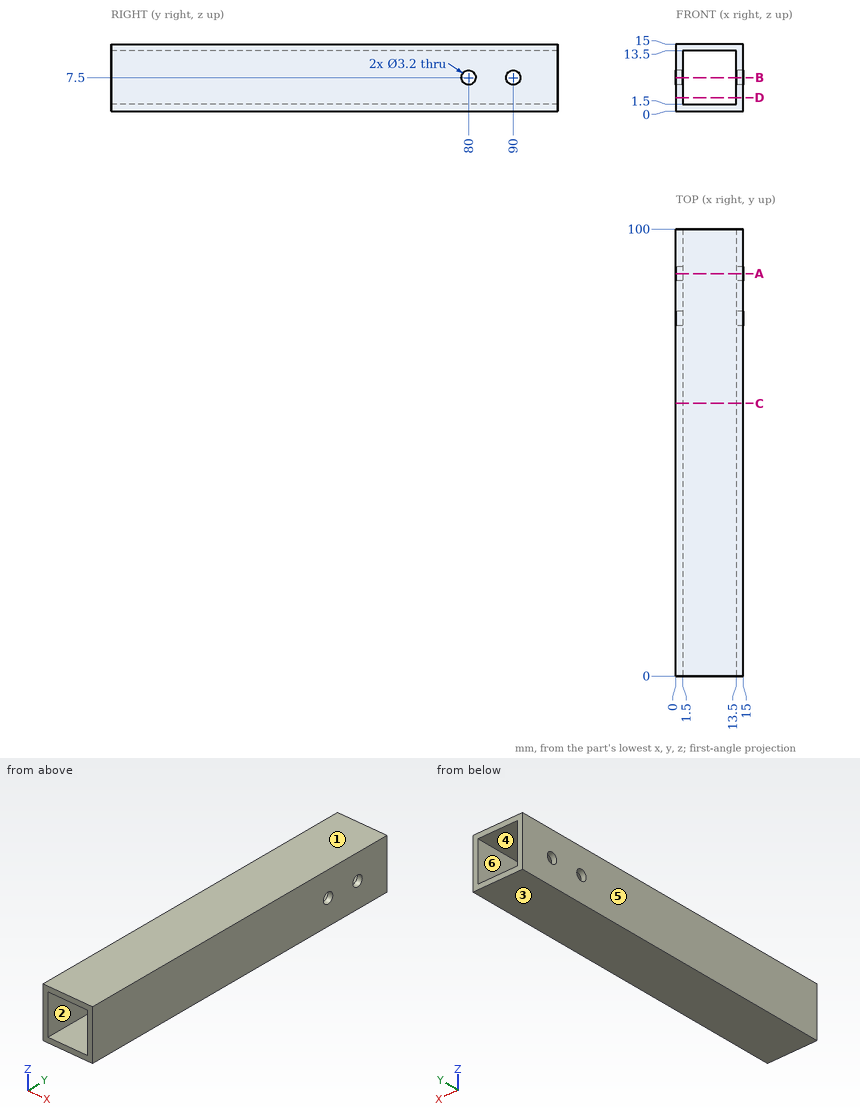
Answer from the drawing. Dimensions are ordinates in mm from the lowest x, y and z of the part. A direction names the side the tool comes from. Round coordinates to 2 decimals unless told otherwise and drop trailing zeros. Order: outer loops, then holes, each group sorted by start corner. A loop starts at its lowest first (then second) coordinate and runs counter-clockwise, first axis right, second up.
1) For the marked faces 1 and 2, determine the directions among +Z, -Z, +X, -X, +Y, -Y from which every point of the face is accessible in a straight line to the end or side of a thin tool.
2) The part is cut by section B-B on z = 7.5. Write down the section's boundary in (x, y), plus the area to 3 significant figures.
3) The part is cut by section C-C on y = 61. Write down the section's boundary in (x, z), plus the area to 3 significant figures.
4) Straight lines are drawn through the part: L1, parallel to Y at x = 0.5, z = 7.5; L2, parallel to Z at x = 6.5, y = 27. For each, find the intervals that lie inside material, in ascending order.
5) The part is cut by section A-A on y = 90. Write down the section's boundary in (x, z), plus the area to 3 significant figures.
6) The mould has two halves that part along Z. Classify the marked faces 3, 4, 5 and 6: released by +Z, released by -Z, zero draft, split by the parting line, or undercut.
7) The part is cut by section D-D on z = 3. Write down the section's boundary in (x, y), plus the area to 3 significant figures.
Resolved:
1. face 1: +Z, +X, -X, +Y, -Y
1. face 2: +Y, -Y
2. outline: (0, 0) - (1.5, 0) - (1.5, 78.4) - (0, 78.4) - close; (0, 81.6) - (1.5, 81.6) - (1.5, 88.4) - (0, 88.4) - close; (0, 91.6) - (1.5, 91.6) - (1.5, 100) - (0, 100) - close; (13.5, 0) - (15, 0) - (15, 78.4) - (13.5, 78.4) - close; (13.5, 81.6) - (15, 81.6) - (15, 88.4) - (13.5, 88.4) - close; (13.5, 91.6) - (15, 91.6) - (15, 100) - (13.5, 100) - close
2. area: 281 mm2
3. outline: (0, 0) - (15, 0) - (15, 15) - (0, 15) - close; hole (1.5, 1.5) - (13.5, 1.5) - (13.5, 13.5) - (1.5, 13.5) - close
3. area: 81.0 mm2
4. L1: y = 0 to 78.4, 81.6 to 88.4, 91.6 to 100
4. L2: z = 0 to 1.5, 13.5 to 15
5. outline: (0, 0) - (15, 0) - (15, 5.9) - (13.5, 5.9) - (13.5, 1.5) - (1.5, 1.5) - (1.5, 5.9) - (0, 5.9) - close; (0, 9.1) - (1.5, 9.1) - (1.5, 13.5) - (13.5, 13.5) - (13.5, 9.1) - (15, 9.1) - (15, 15) - (0, 15) - close
5. area: 71.4 mm2
6. face 3: released by -Z
6. face 4: undercut
6. face 5: zero draft
6. face 6: undercut
7. outline: (0, 0) - (1.5, 0) - (1.5, 100) - (0, 100) - close; (13.5, 0) - (15, 0) - (15, 100) - (13.5, 100) - close
7. area: 300 mm2
